from build123d import *

# Parameters (mm, degrees)
BOSS_EXTRUDE7_DEPTH   = 39
BOSS_EXTRUDE7_2_DEPTH = 39
BOSS_EXTRUDE7_3_DEPTH = 39
BOSS_EXTRUDE7_4_DEPTH = 39
SKETCH1_11_R          = 1.5
BOSS_EXTRUDE8_DEPTH   = 2.5
SKETCH1_12_W          = 67
SKETCH1_12_H          = 5
SKETCH1_12_W_2        = 7
SKETCH1_12_H_2        = 26
BOSS_EXTRUDE9_DEPTH   = 15
SKETCH1_19_R          = 1.5
BOSS_EXTRUDE12_DEPTH  = 37
SKETCH1_20_R          = 1.5
BOSS_EXTRUDE13_DEPTH  = 15
SKETCH4_W             = 13.6
SKETCH4_H             = 36.5
CUT_EXTRUDE2_DEPTH    = 8
SKETCH5_W             = 30
SKETCH5_H             = 10
CUT_EXTRUDE4_DEPTH    = 15


with BuildPart() as part:
    # Sketch1 → Boss-Extrude7 (new body)
    with BuildSketch(Plane(origin=(0, 0, 0), x_dir=(1, 0, 0), z_dir=(0, 1, 0))):
        Polygon((5, 0), (0, 0), (0, 5), (-7, 5), (-7, -5), (5, -5), align=None)
        Polygon((-5.735382907, -1.8), (-4.17653718, 0.9), (-1.058845727, 0.9), (0.5, -1.8), (-1.058845727, -4.5), (-4.17653718, -4.5), align=None, mode=Mode.SUBTRACT)
    extrude(amount=BOSS_EXTRUDE7_DEPTH)



with BuildPart() as body_2:
    # Sketch1 → Boss-Extrude7 2 (new body)
    with BuildSketch(Plane(origin=(0, 0, 0), x_dir=(1, 0, 0), z_dir=(0, 1, 0))):
        Polygon((77, 0), (72, 0), (72, -5), (84, -5), (84, 5), (77, 5), align=None)
        Polygon((81.17653718, 0.9), (82.735382907, -1.8), (81.17653718, -4.5), (78.058845727, -4.5), (76.5, -1.8), (78.058845727, 0.9), align=None, mode=Mode.SUBTRACT)
    extrude(amount=BOSS_EXTRUDE7_2_DEPTH)


with BuildPart() as body_3:
    # Sketch1 → Boss-Extrude7 3 (new body)
    with BuildSketch(Plane(origin=(0, 0, 0), x_dir=(1, 0, 0), z_dir=(0, 1, 0))):
        Polygon((-7, 31), (0, 31), (0, 36), (5, 36), (5, 41), (-7, 41), align=None)
        Polygon((0.5, 37.8), (-1.058845727, 35.1), (-4.17653718, 35.1), (-5.735382907, 37.8), (-4.17653718, 40.5), (-1.058845727, 40.5), align=None, mode=Mode.SUBTRACT)
    extrude(amount=BOSS_EXTRUDE7_3_DEPTH)


with BuildPart() as body_4:
    # Sketch1 → Boss-Extrude7 4 (new body)
    with BuildSketch(Plane(origin=(0, 0, 0), x_dir=(1, 0, 0), z_dir=(0, 1, 0))):
        Polygon((77, 36), (77, 31), (84, 31), (84, 41), (72, 41), (72, 36), align=None)
        Polygon((82.735382907, 37.8), (81.17653718, 35.1), (78.058845727, 35.1), (76.5, 37.8), (78.058845727, 40.5), (81.17653718, 40.5), align=None, mode=Mode.SUBTRACT)
    extrude(amount=BOSS_EXTRUDE7_4_DEPTH)


    add(body_2.part)  # Boss-Extrude8 merges body 2

    add(body_3.part)  # Boss-Extrude8 merges body 3
    # Sketch1_11 → Boss-Extrude8 (add)
    with BuildSketch(Plane(origin=(0, 0, 0), x_dir=(1, 0, 0), z_dir=(0, 1, 0))):
        Polygon((0, 5), (0, 0), (5, 0), (72, 0), (77, 0), (77, 5), (77, 31), (77, 36), (72, 36), (5, 36), (0, 36), (0, 31), align=None)
        with Locations((29, 8.5)):
            Circle(SKETCH1_11_R, mode=Mode.SUBTRACT)
        with Locations((48, 8.5)):
            Circle(SKETCH1_11_R, mode=Mode.SUBTRACT)
        with Locations((29, 27.5)):
            Circle(SKETCH1_11_R, mode=Mode.SUBTRACT)
        with Locations((48, 27.5)):
            Circle(SKETCH1_11_R, mode=Mode.SUBTRACT)
    extrude(amount=BOSS_EXTRUDE8_DEPTH)

    # Sketch1_12 → Boss-Extrude9 (add)
    with BuildSketch(Plane(origin=(0, 0, 0), x_dir=(1, 0, 0), z_dir=(0, 1, 0))):
        with Locations((38.5, -2.5)):
            Rectangle(SKETCH1_12_W, SKETCH1_12_H)
        with Locations((-3.5, 18)):
            Rectangle(SKETCH1_12_W_2, SKETCH1_12_H_2)
        with Locations((38.5, 38.5)):
            Rectangle(SKETCH1_12_W, SKETCH1_12_H)
        with Locations((80.5, 18)):
            Rectangle(SKETCH1_12_W_2, SKETCH1_12_H_2)
    extrude(amount=BOSS_EXTRUDE9_DEPTH)


with BuildPart() as part_1:
    add(part.part)

    add(body_4.part)  # Boss-Extrude12 merges body 4
    # Sketch1_19 → Boss-Extrude12 (add)
    with BuildSketch(Plane(origin=(0, 0, 0), x_dir=(1, 0, 0), z_dir=(0, 1, 0))):
        Polygon((-5.735382907, 37.8), (-4.17653718, 35.1), (-1.058845727, 35.1), (0.5, 37.8), (-1.058845727, 40.5), (-4.17653718, 40.5), align=None)
        with Locations((-2.617691454, 37.9)):
            Circle(SKETCH1_19_R, mode=Mode.SUBTRACT)
        Polygon((-1.058845727, 0.9), (0.5, -1.8), (-1.058845727, -4.5), (-4.17653718, -4.5), (-5.735382907, -1.8), (-4.17653718, 0.9), align=None)
        with Locations((-2.617691454, -1.9)):
            Circle(SKETCH1_19_R, mode=Mode.SUBTRACT)
        Polygon((82.735382907, -1.8), (81.17653718, 0.9), (78.058845727, 0.9), (76.5, -1.8), (78.058845727, -4.5), (81.17653718, -4.5), align=None)
        with Locations((79.617691454, -1.9)):
            Circle(SKETCH1_19_R, mode=Mode.SUBTRACT)
        Polygon((78.058845727, 35.1), (76.5, 37.8), (78.058845727, 40.5), (81.17653718, 40.5), (82.735382907, 37.8), (81.17653718, 35.1), align=None)
        with Locations((79.617691454, 37.9)):
            Circle(SKETCH1_19_R, mode=Mode.SUBTRACT)
    extrude(amount=BOSS_EXTRUDE12_DEPTH)

    # Sketch1_20 → Boss-Extrude13 (add)
    with BuildSketch(Plane(origin=(0, 0, 0), x_dir=(1, 0, 0), z_dir=(0, 1, 0))):
        with Locations((-2.617691454, 37.9)):
            Circle(SKETCH1_20_R)
        with Locations((-2.617691454, -1.9)):
            Circle(SKETCH1_20_R)
        with Locations((79.617691454, -1.9)):
            Circle(SKETCH1_20_R)
        with Locations((79.617691454, 37.9)):
            Circle(SKETCH1_20_R)
    extrude(amount=BOSS_EXTRUDE13_DEPTH)

    # Sketch4 → Cut-Extrude2 (cut, through all)
    with BuildSketch(Plane(origin=(0, 0, 0), x_dir=(0, 0, -1), z_dir=(1, 0, 0))):
        with Locations((8.2, 20.75)):
            Rectangle(SKETCH4_W, SKETCH4_H)
    extrude(amount=-CUT_EXTRUDE2_DEPTH, mode=Mode.SUBTRACT)

    # Sketch5 → Cut-Extrude4 (cut)
    with BuildSketch(Plane.XY.offset(5)):
        with Locations((20, 10)):
            Rectangle(SKETCH5_W, SKETCH5_H)
    extrude(amount=-CUT_EXTRUDE4_DEPTH, mode=Mode.SUBTRACT)


solid = part_1.part
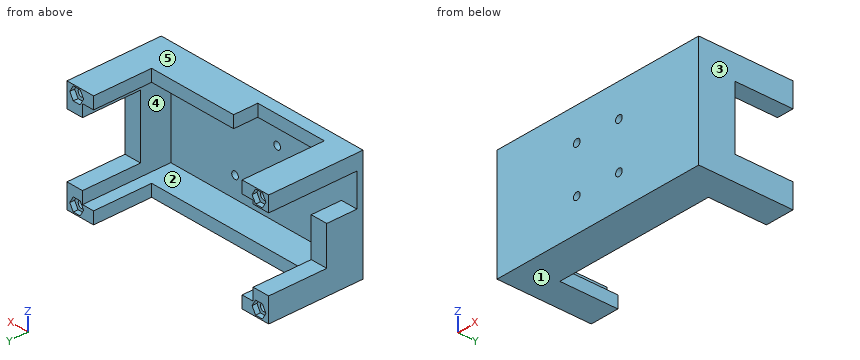
Work out the finished part from the listing and answer in its coordinate system (mm). Face numbers are marked on the shaded views. A direction names the side the tool comes from. Give positions to 0.01 mm unless a question says otherwise; leave off trailing zeros. Write each loop counter-clockwise with the first axis right and the second up, starting at its lowest first coordinate (ties: lowest second). Pieces come first, ordered by that corner, then holes. Notation, with made-up numbers: M 21,-34 L 49,-34 A8 ccw 49,-30 Z; hole C 65.5,-17.5 d4. An arc over 180 degrees is marked long. Answer as CSV lines item,"result".
Q1. A cutting plane is placed at A-A on y = 23.5. Write down the section's boundary in (x, z), plus the area to 3 significant figures.
A:
outline,"M -7,-41 L 5,-41 L 5,-36 L 0,-36 L 0,-31 L -7,-31 Z; M -7,-1.4 L 0,-1.4 L 0,0 L 5,0 L 5,5 L -7,5 Z; M 72,-41 L 84,-41 L 84,-31 L 77,-31 L 77,-36 L 72,-36 Z; M 72,0 L 77,0 L 77,-5 L 84,-5 L 84,5 L 72,5 Z; hole C -2.62,-37.9 d3; hole C -2.62,1.9 d3; hole C 79.62,-37.9 d3; hole C 79.62,1.9 d3"
area,"327 mm²"
Q2. The mould has two halves that part along X. Classify the marked faces 3, 4 and 5: +X half, -X half, draft (parallel to the pull), parting line (faces both ways), or undercut.
A:
face 3,"+X half"
face 4,"undercut"
face 5,"draft"
Q3. Find the intervals of material crossed by probe 1 along Z at (x, y) = (48, 1.5); probe 2 along X at (y, z) = (1.85, -8.5); probe 3 along Z at (x, y) = (51, 5.5), in increasing order. Write a range as [from, to].
A:
probe 1,"z = [-41, -29], [-26, -10], [-7, 5]"
probe 2,"x = [-7, 27.5], [30.5, 46.5], [49.5, 84]"
probe 3,"z = [-41, -36], [0, 5]"
Q4. A tool of negligible diameter and unlimited length cuts with its end or side. For the marked faces 1 and 2, from which of +Z, -Z, +X, -X, +Y, -Y can it reach the whole face along a straight path? Write none if from no direction.
A:
face 1,"-Z, +X, -X, +Y, -Y"
face 2,"+Y"
Q5. A cutting plane is placed at C-C on x = 29. Write down the section's boundary in (y, z), plus the area to 3 significant figures.
A:
outline,"M 0,-41 L 15,-41 L 15,-36 L 2.5,-36 L 2.5,-29 L 0,-29 Z; M 0,-26 L 2.5,-26 L 2.5,-10 L 0,-10 Z; M 0,-7 L 2.5,-7 L 2.5,0 L 5,0 L 5,5 L 0,5 Z"
area,"175 mm²"
Q6. Given P1, Ø1.5, axis at x = -3, z = 1.5, coming from the +Y side; P2, Ø18, axis at x = 28.5, y = 30, coming from the +Z side; P3, Ø3.5, axis at x = 79.62, z = 1.9, coming from the +Y side; P4, Ø1, axis at x = 59, z = -15.5, coming from the +Y side, each flat-ended and moving along its own axis, determine where each tip first touches the part or whether it passes through.
A:
P1,"stops at y = 15"
P2,"passes through"
P3,"stops at y = 37"
P4,"stops at y = 2.5"
Q7. A cutting plane is placed at B-B on z = -8.5. Write down the section's boundary in (x, y), plus the area to 3 significant figures.
A:
outline,"M -7,0 L 27.5,0 L 27.5,2.5 L -7,2.5 Z; M 30.5,0 L 46.5,0 L 46.5,2.5 L 30.5,2.5 Z; M 49.5,0 L 84,0 L 84,15 L 77,15 L 77,2.5 L 49.5,2.5 Z"
area,"300 mm²"
Q8. A cutting plane is placed at D-D on x = 3.5. Write down the section's boundary in (y, z), plus the area to 3 significant figures.
A:
outline,"M 0,-41 L 39,-41 L 39,-36 L 2.5,-36 L 2.5,0 L 39,0 L 39,5 L 0,5 Z"
area,"480 mm²"
